Geometry: see drawing. Coordinates: mm, zero at the bounding-box minimum. A direction names the side the tool comes from. Give positions to 0.01 mm unless a question says otherwise; leave off trailing zeros. Write each loop counter-clockwise with the first axis right and the second up, starting at its lowest first coordinate (ties: lowest second). Pieces come first, ordered by that corner, then holes. Notation, with made-up numbers: (-37.5, -19.5) - (21.5, -19.5) arc R20 cw to (21.5, -13.5) - close; hole circle Ø9 at (31, 63.5). An arc over 180 degrees is marked (long way). Use CSV: the item, a comma, the result in double quotes. Start each with the question number.
(1) Section D-D on y = 21.5. Output: boundary loops of the cut face in (x, z) (3 decimals).
(2) Draft query along X for the marked faces 1, 2 and 3. Return one class per face: released by +X, released by -X, zero draft, split by the parting line, or undercut.
(3) First-contact query: pin 1 Ø5 at (x, y) = (14.5, 6) entering from -Z; pin 2 Ø1.5 at (x, y) = (7.5, 22.5) entering from +Z (3 decimals). Flat tips, straight axial feed; report the tip coordinate or a pass-through.
(4) Reachability of the marked faces 4 and 5 from +Z, -Z, +X, -X, +Y, -Y: full face, straight path, thin tool, end or side. Return the list, or none.
(5) Section A-A on z = 2.6. Output: boundary loops of the cut face in (x, y).
(6) Line query: probe 1 along Y at (x, z) = (5.08, 2.4); probe 2 along X at (y, z) = (20.32, 1.4); probe 3 along Y at (x, z) = (6.75, 0.5). Output: solid intervals per line, ascending. Write a range as [from, to].
(7) Section C-C on y = 4.5. Output: boundary loops of the cut face in (x, z) (3 decimals).
(8) Section B-B on x = 5.08. Output: boundary loops of the cut face in (y, z) (3 decimals).
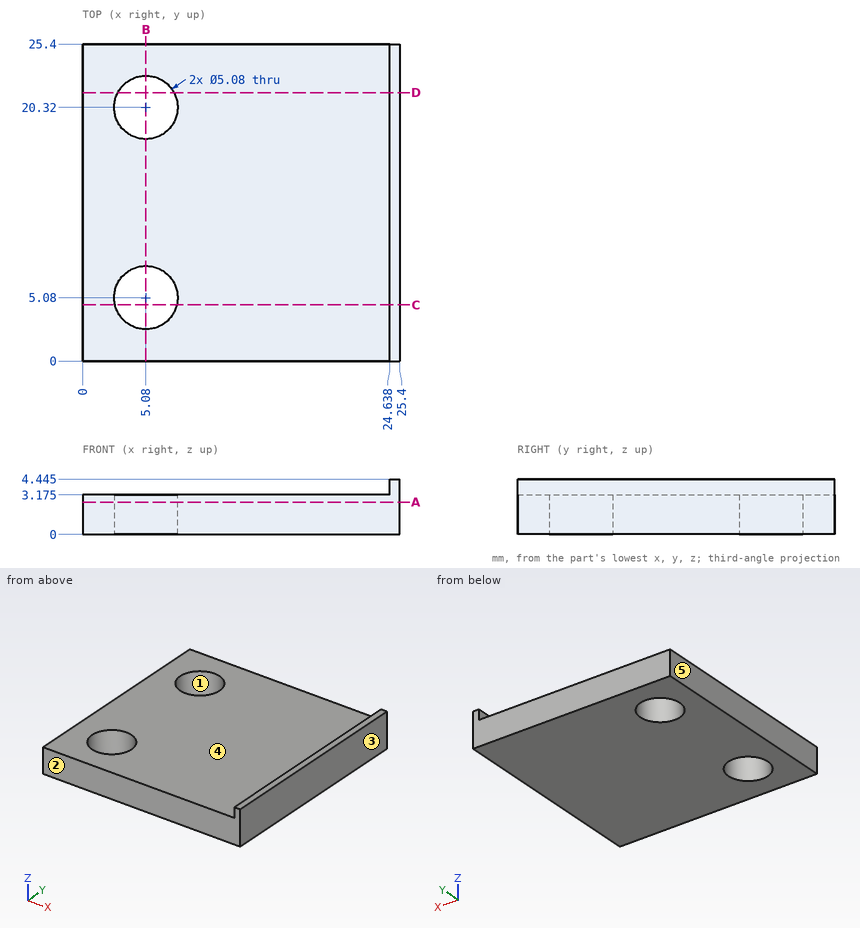
Check values:
1,outline,"(0, 0) - (2.831, 0) - (2.831, 3.175) - (0, 3.175) - close; (7.329, 0) - (25.4, 0) - (25.4, 4.445) - (24.638, 4.445) - (24.638, 3.175) - (7.329, 3.175) - close"
2,face 1,"undercut"
2,face 2,"zero draft"
2,face 3,"released by +X"
3,pin 1,"stops at z = 0"
3,pin 2,"stops at z = 3.175"
4,face 4,"+Z, -X, +Y, -Y"
4,face 5,"+Z, -Z, -X, +Y, -Y"
5,outline,"(0, 0) - (25.4, 0) - (25.4, 25.4) - (0, 25.4) - close; hole circle Ø5.08 at (5.08, 5.08); hole circle Ø5.08 at (5.08, 20.32)"
6,probe 1,"y = [0, 2.54], [7.62, 17.78], [22.86, 25.4]"
6,probe 2,"x = [0, 2.54], [7.62, 25.4]"
6,probe 3,"y = [0, 3.17], [6.99, 18.41], [22.23, 25.4]"
7,outline,"(0, 0) - (2.607, 0) - (2.607, 3.175) - (0, 3.175) - close; (7.553, 0) - (25.4, 0) - (25.4, 4.445) - (24.638, 4.445) - (24.638, 3.175) - (7.553, 3.175) - close"
8,outline,"(0, 0) - (2.54, 0) - (2.54, 3.175) - (0, 3.175) - close; (7.62, 0) - (17.78, 0) - (17.78, 3.175) - (7.62, 3.175) - close; (22.86, 0) - (25.4, 0) - (25.4, 3.175) - (22.86, 3.175) - close"
